The listing builds one solid part. Answer for the finished solid, in the listing's coordinates (mm). A direction names the side the tool comes from. Give positions to 0.01 mm unless a question says otherwise; leave off trailing zeros. Write each loop counter-clockwise with the first axis right and the second up, starting at its lowest first coordinate (ties: lowest second). Pieces come first, ordered by that corner, then holes. Notation, with made-up numbers: (67.5, -12.5) - (117.5, -12.5) arc R24 cw to (117.5, 14.5) - close; hole circle Ø8 at (13.25, 80.5). An arc over 180 degrees is marked (long way). Write each question's results on one line, items separated by ' | '. Start each with the question number.
Q1. Section D-D (z = -33) is taken. Determine the outline of the cut face in (x, y), plus the area to 3 significant figures.
Q2. For a pull along Y with two mould halves and no side action, classify faces 1 (the face through (-2.44, 0, 2)), 2 (the face through (3, 0, -19)), 3 (the face through (0, 0, -36)) as pulls with the +Y half, pulls with the -Y half, needs draft (parallel to the pull), parting line crosses it, or undercut.
Q3. Section C-C (x = 0.75) is taken. Determine the outline of the cut face in (y, z).
Q4. Section A-A (z = 1) is taken. Determine the outline of the cut face in (x, y), plus the area to 3 significant figures.
Q5. Flat-ended cylindrical pins translate along their axes: pin 1 Ø3 at (y, z) = (3.5, -2) entering from -X; pin 2 Ø5 at (x, z) = (-2.5, -20.5) entering from -Y; pin 3 Ø2 at (y, z) = (-1.5, -25) entering from -X. Find the tip coordinate at first contact, or state that the pin passes through.
Q6. For faces 4 (the face through (2.44, 0, 2)), 5 (the face through (2, -2, 4)), 6 (the face through (-1, -3, -2)), determine the directions among +Z, -Z, +X, -X, +Y, -Y from which every point of the face is accessible in a straight line to the end or side of a thin tool.
Q7. Find the intervals of material crossed by probe 1 along Z at (x, y) = (3.25, 2.5); probe 2 along Y at (x, z) = (0, -15); probe 3 along Z at (x, y) = (-2, -1), in increasing order.
Q8. Section B-B (y = 0) is taken. Determine the outline of the cut face in (x, z), plus the area to 3 significant figures.
```python
from build123d import *

# Parameters (mm, degrees)
SKETCH1_R           = 4.5
BOSS_EXTRUDE1_DEPTH = 4
SKETCH2_R           = 4.5
BOSS_EXTRUDE2_DEPTH = 2
SKETCH3_R           = 3
BOSS_EXTRUDE3_DEPTH = 34


with BuildPart() as part:
    # Sketch1 → Boss-Extrude1 (new body)
    with BuildSketch(Plane.XY):
        Circle(SKETCH1_R)
        Polygon((0, 2.817703613), (-2.440202909, 1.408851806), (-2.440202909, -1.408851806), (0, -2.817703613), (2.440202909, -1.408851806), (2.440202909, 1.408851806), align=None, mode=Mode.SUBTRACT)
    extrude(amount=BOSS_EXTRUDE1_DEPTH)

    # Sketch2 → Boss-Extrude2 (add)
    with BuildSketch(Plane(origin=(0, 0, 0), x_dir=(-1, 0, 0), z_dir=(0, 0, -1))):
        Circle(SKETCH2_R)
    extrude(amount=BOSS_EXTRUDE2_DEPTH)

    # Sketch3 → Boss-Extrude3 (add)
    with BuildSketch(Plane(origin=(0, 0, -2), x_dir=(-1, 0, 0), z_dir=(0, 0, -1))):
        Circle(SKETCH3_R)
    extrude(amount=BOSS_EXTRUDE3_DEPTH)


solid = part.part
```
Answers below:
1) outline: circle Ø6 at (0, 0) | area: 28.3 mm2
2) face 1: undercut | face 2: parting line crosses it | face 3: needs draft
3) outline: (-4.44, -2) - (-2.9, -2) - (-2.9, -36) - (2.9, -36) - (2.9, -2) - (4.44, -2) - (4.44, 4) - (2.38, 4) - (2.38, 0) - (-2.38, 0) - (-2.38, 4) - (-4.44, 4) - close
4) outline: circle Ø9 at (0, 0); hole (-2.44, -1.41) - (0, -2.82) - (2.44, -1.41) - (2.44, 1.41) - (0, 2.82) - (-2.44, 1.41) - close | area: 43.0 mm2
5) pin 1: stops at x = -4.03 | pin 2: stops at y = -3 | pin 3: stops at x = -2.96
6) face 4: +Z | face 5: +Z, +X, -X, +Y, -Y | face 6: -Z
7) probe 1: z = -2 to 4 | probe 2: y = -3 to 3 | probe 3: z = -36 to 0
8) outline: (-4.5, -2) - (-3, -2) - (-3, -36) - (3, -36) - (3, -2) - (4.5, -2) - (4.5, 4) - (2.44, 4) - (2.44, 0) - (-2.44, 0) - (-2.44, 4) - (-4.5, 4) - close | area: 238 mm2
